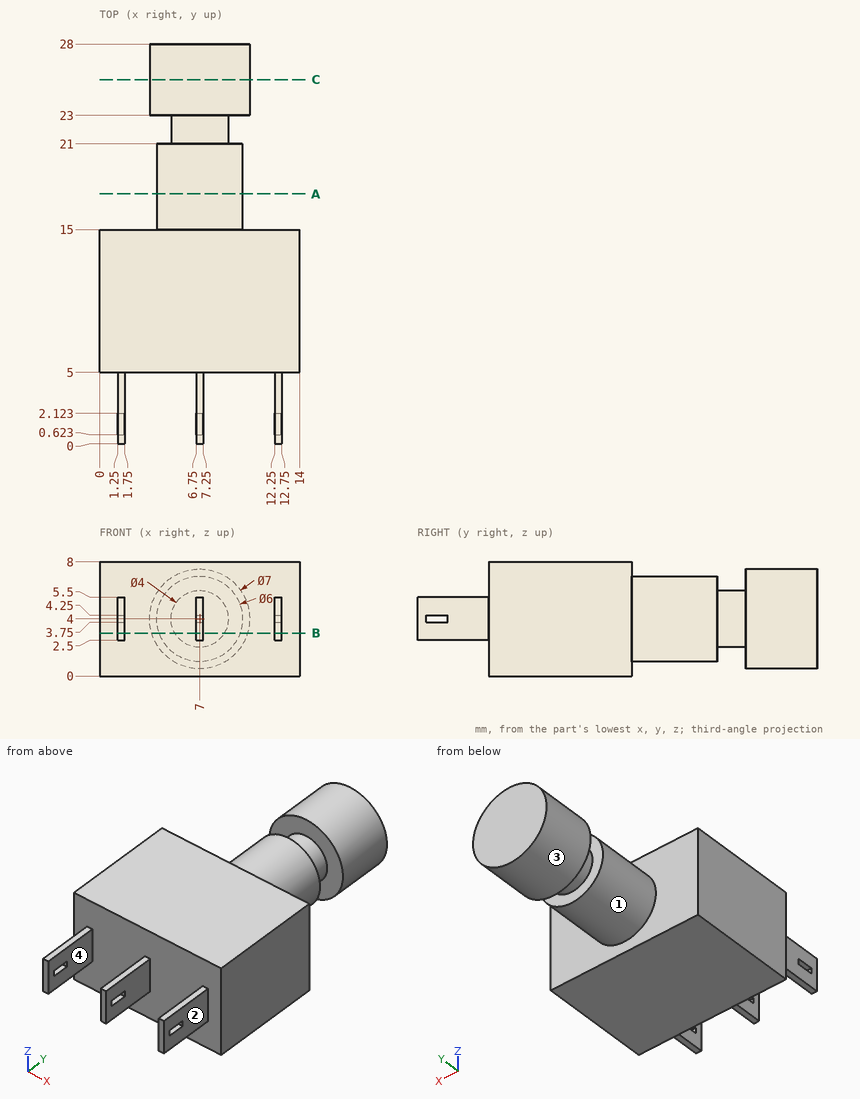
Here's the drawing with two shaded views (mm, measured from the low corner). I have some questions. A direction names the side the tool comes from. Give positions to 0.01 mm unless a question says otherwise; leave off trailing zeros. Loops run counter-clockwise (first coordinate to the right, second up) from the corner with the lowest first, then second, coordinate; pieces in that order, holes last. Notation, with made-up numbers: M 57.5,83.5 L 100.5,83.5 A21 ccw 100.5,108.5 Z; hole C 45.5,25.5 d11. An arc over 180 degrees is marked long. One line per item, written item: value. Start each with the question number.
1) I'm going to push flat-ended pins straight in: pin 1 (0.6 mm diameter, centred on x = 1.5, y = 1, fed in from +Z); pin 2 (1.5 mm diameter, centred on y = 2, z = 4, fed in from +X); pin 3 (0.6 mm diameter, centred on x = 1.5, y = 2.5, fed in from -Z); pin 4 (1 mm diameter, centred on y = 3.5, z = 1.5, fed in from +X). Where does each tip first touch, or does it pass through?
2) If we section it at B-B, the plane z = 3: Write out the boundary of the cut face in (x, y), and give its area (3 significant figures).
3) If I drill on line 1 (X direction, y = 4, z = 5.25); line 2 (Y direction, x = 5.75, z = 6); line 3 (Y direction, x = 10.5, z = 0.5), over which ranges is the centre line in solid material (lowest first)? Write a range as [from, to].
4) If we section it at A-A, the plane y = 17.5: Write out the boundary of the cut face in (x, z).
5) On a 3-axis mill with a long thin cutter (end or side, diameter ignored), from which of +Z, -Z, +X, -X, +Y, -Y can I reach the whole of each face in a straight line? I mean the marked faces 1, 2, 3 and 4. Say none if no direction works.
6) If we section it at C-C, the plane y = 25.5: Write out the boundary of the cut face in (x, z).
Completed:
1. pin 1: stops at z = 5.5
1. pin 2: stops at x = 12.75
1. pin 3: stops at z = 2.5
1. pin 4: passes through
2. outline: M 0,5 L 1.25,5 L 1.25,0 L 1.75,0 L 1.75,5 L 6.75,5 L 6.75,0 L 7.25,0 L 7.25,5 L 12.25,5 L 12.25,0 L 12.75,0 L 12.75,5 L 14,5 L 14,15 L 9.83,15 L 9.83,21 L 8.73,21 L 8.73,23 L 10.35,23 L 10.35,28 L 3.65,28 L 3.65,23 L 5.27,23 L 5.27,21 L 4.17,21 L 4.17,15 L 0,15 Z
2. area: 222 mm^2
3. line 1: x = [1.25, 1.75], [6.75, 7.25], [12.25, 12.75]
3. line 2: y = [5, 21], [23, 28]
3. line 3: y = [5, 15]
4. outline: C 7,4 d6
5. face 1: none
5. face 2: +Z, -Z, +X, -Y
5. face 3: +Y
5. face 4: +Z, -Z, -Y
6. outline: C 7,4 d7
